Could you check a few things on this drawing? It's one solid part, dimensions in mm from its lowest x, y, z. Give positions to 0.01 mm unless a question says otherwise; leave off trailing zeros. Order: outer loops, then holes, each group sorted by start corner. A loop starts at its lowest first (then second) coordinate and runs counter-clockwise, first axis right, second up. Notation, with made-up numbers: M 24,40.25 L 51,40.25 A24 cw 51,74.25 Z; hole C 19,38 d3. An arc over 180 degrees is marked long. Use CSV: the item, a comma, the result in double quotes. Start each with the question number.
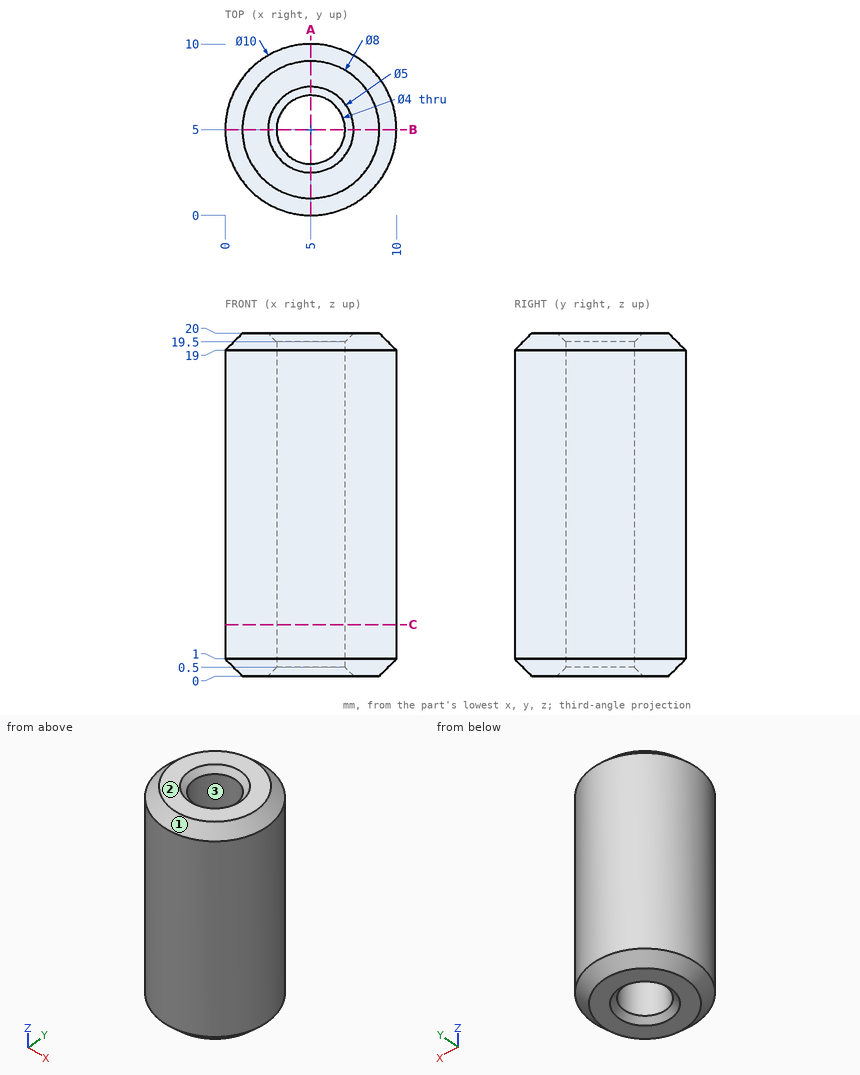
Q1. For P1, Ø1.5, axis at x = 4.5, y = 4, coming from the +Z side; P2, Ø4, axis at y = 6, z = 8.5, coming from the +X side; P3, Ø2, axis at x = 7.5, z = 14, coming from the -Y side; P4, Ø5, axis at y = 8.5, z = 3, coming from the -X side, each with a flat end and sliding along its axis, tell me the tip position at first contact or that it passes through.
Q2. Imagine slicing it at A-A, the plane x = 5. Please give me the cut outline in (y, z), then the cut area to 4 significant figures.
Q3. We'd pull the mould along Y, two halves only. Please class the marked faces 1, 2 and 3: pulls with the +Y half, pulls with the -Y half, needs draft (parallel to the pull), parting line crosses it, or undercut.
Q4. Imagine slicing it at C-C, the plane z = 3. Please give me the cut outline in (x, y).
Q5. I need wall thicknesses on line 1 (Y direction, x = 5, z = 11); line 2 (Y direction, x = 6.25, z = 16.75); line 3 (X direction, y = 5.75, z = 2). Which ranges of each line are inside material? Lowest first, please. Write a range as [from, to].
Reply:
1,P1,"passes through"
1,P2,"stops at x = 10"
1,P3,"stops at y = 0.23"
1,P4,"stops at x = 0.1"
2,outline,"M 0,1 L 1,0 L 2.5,0 L 3,0.5 L 3,19.5 L 2.5,20 L 1,20 L 0,19 Z; M 7,0.5 L 7.5,0 L 9,0 L 10,1 L 10,19 L 9,20 L 7.5,20 L 7,19.5 Z"
2,area,"117.5 mm^2"
3,face 1,"parting line crosses it"
3,face 2,"needs draft"
3,face 3,"undercut"
4,outline,"C 5,5 d10; hole C 5,5 d4"
5,line 1,"y = [0, 3], [7, 10]"
5,line 2,"y = [0.16, 3.44], [6.56, 9.84]"
5,line 3,"x = [0.06, 3.15], [6.85, 9.94]"
